```python
from build123d import *

# Parameters (mm, degrees)
ESQUISSE1_W             = 152.4
ESQUISSE1_H             = 12.7
BOSS_EXTRU_1_DEPTH      = 6.35
ESQUISSE2_R             = 2.38125
ESQUISSE2_W             = 3.367596046
ESQUISSE2_H             = 3.367596046
ESQUISSE2_W_2           = 3.167596046
ESQUISSE2_H_2           = 3.167596046
ENL_V_MAT_EXTRU_1_DEPTH = 154.060029074
SKETCH1_W               = 14.17076538
SKETCH1_H               = 3.495000122
CUT_REVOLVE1_ANGLE      = 180
SKETCH2_W               = 3.495000122
SKETCH2_H               = 3.683
CUT_EXTRUDE1_DEPTH      = 154.060029074


with BuildPart() as part:
    # Esquisse1 → Boss.-Extru.1 (new body)
    with BuildSketch(Plane.XY):
        with Locations((-76.2, 6.35)):
            Rectangle(ESQUISSE1_W, ESQUISSE1_H)
    extrude(amount=-BOSS_EXTRU_1_DEPTH)

    # Esquisse2 → Enl_v. mat.-Extru.1 (cut, through all)
    # profile 1 of 8: a face of its own
    with BuildSketch(Plane.XY):
        with Locations((-146.05, 6.35)):
            Circle(ESQUISSE2_R)
    # profile 2 of 8: a face of its own
    with BuildSketch(Plane.XY):
        with Locations((-76.2, 6.35)):
            Circle(ESQUISSE2_R)
    # profile 3 of 8: a face of its own
    with BuildSketch(Plane.XY):
        with BuildLine():
            Line((0, 12.7), (-6.35, 12.7))
            ThreePointArc((-6.35, 12.7), (-1.859871939, 10.840128061), (0, 6.35))
            Line((0, 6.35), (0, 12.7))
        make_face()
    # profile 4 of 8: a face of its own
    with BuildSketch(Plane.XY):
        with BuildLine():
            Line((0, 0), (0, 6.35))
            ThreePointArc((0, 6.35), (-1.859871939, 1.859871939), (-6.35, 0))
            Line((-6.35, 0), (0, 0))
        make_face()
    # profile 5 of 8: a face of its own
    with BuildSketch(Plane.XY):
        with BuildLine():
            ThreePointArc((-152.4, 6.35), (-150.540128061, 10.840128061), (-146.05, 12.7))
            Line((-146.05, 12.7), (-152.4, 12.7))
            Line((-152.4, 12.7), (-152.4, 6.35))
        make_face()
    # profile 6 of 8: a face of its own
    with BuildSketch(Plane.XY):
        with BuildLine():
            ThreePointArc((-146.05, 0), (-150.540128061, 1.859871939), (-152.4, 6.35))
            Line((-152.4, 6.35), (-152.4, 0))
            Line((-152.4, 0), (-146.05, 0))
        make_face()
    # profile 7 of 8: a face of its own
    with BuildSketch(Plane.XY):
        with Locations((-6.35, 6.35)):
            Rectangle(ESQUISSE2_W, ESQUISSE2_H)
        with Locations((-6.35, 6.35)):
            Rectangle(ESQUISSE2_W_2, ESQUISSE2_H_2, mode=Mode.SUBTRACT)
    # profile 8 of 8: a face of its own
    with BuildSketch(Plane.XY):
        with Locations((-6.35, 6.35)):
            Rectangle(ESQUISSE2_W_2, ESQUISSE2_H_2)
    extrude(amount=-ENL_V_MAT_EXTRU_1_DEPTH, mode=Mode.SUBTRACT)

    # Sketch1 → Cut-Revolve1 (revolve, symmetric, cut)
    with BuildSketch(Plane(origin=(0, 6.35, 0), x_dir=(1, 0, 0), z_dir=(0, 1, 0))) as cut_revolve1_sk:
        Polygon((-150.5585, 1.427499939), (-152.4, 1.427499939), (-152.4, 4.922500061), (-150.5585, 4.922500061), (-148.717, 4.922500061), (-148.717, 1.427499939), align=None)
        with Locations((-159.48538269, 3.175)):
            Rectangle(SKETCH1_W, SKETCH1_H)
    cut_revolve1 = revolve(axis=Axis((-146.05, 6.35, -6.35), (0, 0, 1)), revolution_arc=CUT_REVOLVE1_ANGLE / 2, mode=Mode.SUBTRACT)
    cut_revolve1 = cut_revolve1 + revolve(cut_revolve1_sk.sketch, axis=Axis((-146.05, 6.35, -6.35), (0, 0, -1)), revolution_arc=CUT_REVOLVE1_ANGLE / 2, mode=Mode.SUBTRACT)

    # Mirror1: Cut-Revolve1 across plane
    add(cut_revolve1.mirror(Plane(origin=(-76.2, 0, 0), x_dir=(0, 0, 1), z_dir=(1, 0, 0))), mode=Mode.SUBTRACT)

    # Sketch2 → Cut-Extrude1 (cut, through all)
    with BuildSketch(Plane(origin=(0, 0, 0), x_dir=(0, 0, -1), z_dir=(1, 0, 0))):
        with Locations((3.175, 10.8585)):
            Rectangle(SKETCH2_W, SKETCH2_H)
    cut_extrude1 = extrude(amount=-CUT_EXTRUDE1_DEPTH, mode=Mode.SUBTRACT)

    # Mirror2: Cut-Extrude1 across plane
    add(cut_extrude1.mirror(Plane.ZX.offset(6.35)), mode=Mode.SUBTRACT)


solid = part.part
```
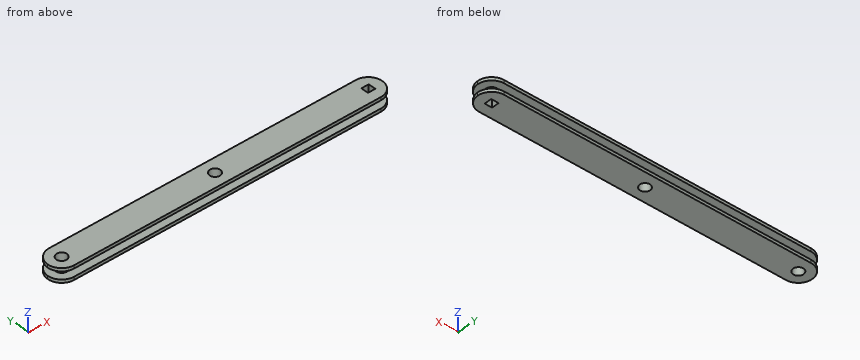
Geometry: final body of the model. Coordinates: model frame, mm. Coordinates: 2 decimals unless noted, no trailing zeros. Order: outer loops, then holes, each group sorted by start corner. A loop starts at its lowest first (then second) coordinate and runs counter-clockwise, first axis right, second up. Notation, with made-up numbers: (15, -16.5) -> (28, -16.5) arc R25 ccw to (28, 8.5) -> close; hole circle Ø4 at (-34.5, 57.25). An arc over 180 degrees is marked (long way). Use CSV: the item, a comma, the result in double quotes.
1) Section C-C on y = 10.25. Output: boundary loops of the cut face in (x, z), then the cut area to 3 significant figures.
Findings:
outline,"(-151.06, -6.35) -> (-1.34, -6.35) -> (-1.34, -4.92) -> (-151.06, -4.92) -> close; (-151.06, -1.43) -> (-1.34, -1.43) -> (-1.34, 0) -> (-151.06, 0) -> close"
area,"427 mm^2"
2) Section B-B on z = -3.75. Output: boundary loops of the cut face in (x, y), then the cut area to 3 significant figures.
Findings:
outline,"(-146.05, 3.68) -> (-6.35, 3.68) arc R2.67 ccw to (-6.35, 9.02) -> (-146.05, 9.02) arc R2.67 ccw to start; hole circle Ø4.76 at (-146.05, 6.35); hole circle Ø4.76 at (-76.2, 6.35); hole (-8.03, 4.67) -> (-4.67, 4.67) -> (-4.67, 8.03) -> (-8.03, 8.03) -> close"
area,"721 mm^2"
3) Section A-A on x = -76.2. Output: boundary loops of the cut face in (y, z).
Findings:
outline,"(0, -6.35) -> (3.97, -6.35) -> (3.97, 0) -> (0, 0) -> (0, -1.43) -> (3.68, -1.43) -> (3.68, -4.92) -> (0, -4.92) -> close; (8.73, -6.35) -> (12.7, -6.35) -> (12.7, -4.92) -> (9.02, -4.92) -> (9.02, -1.43) -> (12.7, -1.43) -> (12.7, 0) -> (8.73, 0) -> close"
4) Line query: line 1 (Y direction, x = -76.2, z = -3); line 2 (X direction, y = 6, z = -5.25); line 3 (Z direction, x = -135.5, y = 10.5). Output: solid intervals per line, ascending.
Findings:
line 1,"y = 3.68 to 3.97, 8.73 to 9.02"
line 2,"x = -152.39 to -148.41, -143.69 to -78.56, -73.84 to -8.03, -4.67 to -0.01"
line 3,"z = -6.35 to -4.92, -1.43 to 0"
5) Pin query (flat end, axial travel): pin 1 Ø2.5 at (x, z) = (-6.5, -3.5) entering from +Y; pin 2 Ø3 at (x, z) = (-91.5, -3.5) entering from -Y; pin 3 Ø1.7 at (y, z) = (5.5, -3.5) entering from -X; pin 4 Ø3 at (y, z) = (9.5, -1.5) entering from +X. Return the tip coordinate at first contact, or that it passes through.
Findings:
pin 1,"stops at y = 9.02"
pin 2,"stops at y = 0"
pin 3,"stops at x = -148.72"
pin 4,"stops at x = -0.22"
6) Section D-D on x = -43. Output: boundary loops of the cut face in (y, z).
Findings:
outline,"(0, -6.35) -> (12.7, -6.35) -> (12.7, -4.92) -> (9.02, -4.92) -> (9.02, -1.43) -> (12.7, -1.43) -> (12.7, 0) -> (0, 0) -> (0, -1.43) -> (3.68, -1.43) -> (3.68, -4.92) -> (0, -4.92) -> close"
